from build123d import *

# Parameters (mm, degrees)
BOSS_EXTRUDE4_DEPTH = 200
CUT_EXTRUDE3_START  = -150
CUT_EXTRUDE3_DEPTH  = 150
SKETCH6_R           = 22.5
CUT_EXTRUDE5_DEPTH  = 120
SKETCH7_R           = 32.5
CUT_EXTRUDE6_DEPTH  = 80
FILLET2_R           = 4
SKETCH8_W           = 40
SKETCH8_H           = 40
CUT_EXTRUDE7_DEPTH  = 18
FILLET3_R           = 5
SKETCH10_W          = 10
SKETCH10_H          = 40
CUT_EXTRUDE9_DEPTH  = 69
SKETCH11_R          = 5
CUT_EXTRUDE10_DEPTH = 10


with BuildPart() as part:
    # Sketch1 → Boss-Extrude4 (new body)
    with BuildSketch(Plane(origin=(0, 0, 0), x_dir=(1, 0, 0), z_dir=(0, 1, 0))):
        with BuildLine():
            Line((0, 50), (-25, 50))
            Line((-25, 50), (-25, 31.224990005))
            ThreePointArc((-25, 31.224990005), (0, -40.00000001), (25, 31.224990005))
            Line((25, 31.224990005), (25, 50))
            Line((25, 50), (0, 50))
        make_face()
    extrude(amount=-BOSS_EXTRUDE4_DEPTH)

    # Sketch5 → Cut-Extrude3 (cut)
    with BuildSketch(Plane.XZ.offset(200).offset(CUT_EXTRUDE3_START)):
        with BuildLine():
            Line((-25, -31.224990005), (-25, -50))
            Line((-25, -50), (25, -50))
            Line((25, -50), (25, -31.224990005))
            ThreePointArc((25, -31.224990005), (0, -40.00000001), (-25, -31.224990005))
        make_face()
    extrude(amount=CUT_EXTRUDE3_DEPTH, mode=Mode.SUBTRACT)

    # Sketch6 → Cut-Extrude5 (cut)
    with BuildSketch(Plane(origin=(0, 0, 0), x_dir=(1, 0, 0), z_dir=(0, 1, 0))):
        with Locations(Location((0, 0, 0), (0, 0, 270))):
            Circle(SKETCH6_R)
    extrude(amount=-CUT_EXTRUDE5_DEPTH, mode=Mode.SUBTRACT)

    # Sketch7 → Cut-Extrude6 (cut)
    with BuildSketch(Plane.XZ.offset(200)):
        with Locations(Location((0, 0, 0), (0, 0, 270))):
            Circle(SKETCH7_R)
    extrude(amount=-CUT_EXTRUDE6_DEPTH, mode=Mode.SUBTRACT)

    # Fillet2
    fillet2_edges = [part.edges().sort_by_distance(p)[0] for p in [
        (0, -120, 32.5),
    ]]
    fillet(fillet2_edges, radius=FILLET2_R)

    # Sketch8 → Cut-Extrude7 (cut)
    with BuildSketch(Plane(origin=(0, 0, -50), x_dir=(-1, 0, 0), z_dir=(0, 0, -1))):
        with Locations((0, -25)):
            Rectangle(SKETCH8_W, SKETCH8_H)
    extrude(amount=-CUT_EXTRUDE7_DEPTH, mode=Mode.SUBTRACT)

    # Fillet3
    fillet3_edges = [part.edges().sort_by_distance(p)[0] for p in [
        (20, -45, -41),
        (20, -5, -41),
        (-20, -5, -41),
        (-20, -45, -41),
    ]]
    fillet(fillet3_edges, radius=FILLET3_R)

    # Sketch10 → Cut-Extrude9 (cut)
    with BuildSketch(Plane(origin=(0, 0, 0), x_dir=(0, 0, -1), z_dir=(1, 0, 0))):
        with Locations((0, -165)):
            Rectangle(SKETCH10_W, SKETCH10_H)
        with BuildLine():
            Line((5, -145), (-5, -145))
            ThreePointArc((-5, -145), (0, -140), (5, -145))
        make_face()
        with BuildLine():
            ThreePointArc((5, -185), (0, -190), (-5, -185))
            Line((-5, -185), (5, -185))
        make_face()
    extrude(amount=CUT_EXTRUDE9_DEPTH, mode=Mode.SUBTRACT)

    # Sketch11 → Cut-Extrude10 (cut)
    with BuildSketch(Plane(origin=(0, 0, 0), x_dir=(1, 0, 0), z_dir=(0, 1, 0))):
        with Locations(Location((30, 0, 0), (0, 0, 270))):
            Circle(SKETCH11_R)
        with Locations(Location((21.213203436, -21.213203436, 0), (0, 0, 270))):
            Circle(SKETCH11_R)
        with Locations(Location((0, -30, 0), (0, 0, 270))):
            Circle(SKETCH11_R)
        with Locations(Location((-21.213203436, -21.213203436, 0), (0, 0, 270))):
            Circle(SKETCH11_R)
        with Locations(Location((-30, 0, 0), (0, 0, 270))):
            Circle(SKETCH11_R)
        with Locations(Location((-21.213203436, 21.213203436, 0), (0, 0, 270))):
            Circle(SKETCH11_R)
        with Locations(Location((0, 30, 0), (0, 0, 270))):
            Circle(SKETCH11_R)
        with Locations(Location((21.213203436, 21.213203436, 0), (0, 0, 270))):
            Circle(SKETCH11_R)
    extrude(amount=-CUT_EXTRUDE10_DEPTH, mode=Mode.SUBTRACT)


solid = part.part
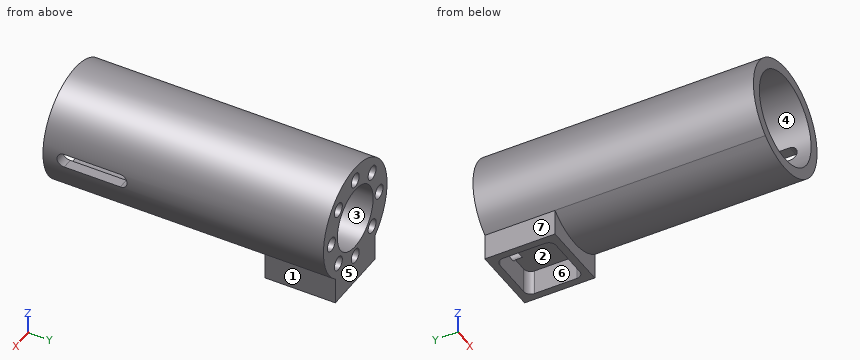
Input: part model. Units: mm. Frame: model coordinates. Face numbers are marked on the shaded views. A direction names the side the tool comes from. Coordinates: 2 decimals unless noted, no trailing zeros. Write each loop counter-clockwise with the first axis right and the second up, starting at its lowest first coordinate (ties: lowest second). Pieces come first, ordered by that corner, then holes. Notation, with made-up numbers: M 79,1 L 105,1 A17 ccw 105,21 Z; hole C 33.25,-7.5 d4. An arc over 180 degrees is marked long. Answer as a JSON object with one key per item and string values. Group by question number.
(1) Ray query, line 1 along X through (y, z) = (-5, 0); line 2 along Y through (x, z) = (25.5, 10); line 3 along Z through (x, y) = (-0.5, -90). Return the intervals inside material, ascending. Write a range as [from, to].
(2) Section D-D on y = -92.5. Output: boundary loops of the cut face in (x, z) (3 decimals).
(3) Contact query for flat-ended pins moving along their axis: P1, Ø6, axis at x = -30, z = 0, coming from the +Y side; P2, Ø1.5, axis at y = -93.5, z = 13, coming from the +X side; P3, Ø4, axis at x = 34.5, y = -169, coming from the -Z side. Output: stop coordinate, or through.
(4) Section C-C on y = -153.5. Output: boundary loops of the cut face in (x, z) (3 decimals).
(5) Section B-B on y = -21.5. Output: boundary loops of the cut face in (x, z) (3 decimals).
(6) Set-up query: the marked faces 1, 2, 3 and 4. Return all of +Z, -Z, +X, -X, +Y, -Y with unobstructed straight access to the full face (end or side cutting, diameter ignored); none if empty.
(7) Section A-A on z = 0. Output: boundary loops of the cut face in (x, y), plus the area to 3 significant figures.
(8) Mould query, pull axis Y, two halves, no side actions, for the marked faces 5, 6 and 7. Classes: pulls with the +Y half, pulls with the -Y half, needs draft (parallel to the pull), parting line crosses it, or undercut.
Result set:
{
 "1": {"line 1": "x = [-40, -35], [-25, -22.5], [22.5, 25], [35, 40]", "line 2": "y = [-120, 0]", "line 3": "z = [-40, -22.49], [22.49, 40]"},
 "2": {"outline": "C 0,0 d80; hole C 0,0 d45"},
 "3": {"P1": "stops at y = -10", "P2": "stops at x = 38.08", "P3": "stops at z = -23.32"},
 "4": {"outline": "M 32.113,-5 A32.5 cw long 32.113,5 L 39.686,5 A40 ccw long 39.686,-5 Z"},
 "5": {"outline": "M -25,-50 L -20,-50 L -20,-32 L 20,-32 L 20,-50 L 25,-50 L 25,-31.225 A40 ccw long -25,-31.225 Z; hole C 0,0 d45"},
 "6": {"face 1": "-Z, +X, +Y, -Y", "face 2": "-Z", "face 3": "+Y, -Y", "face 4": "-Y"},
 "7": {"outline": "M -40,-200 L -32.5,-200 L -32.5,-124 A4 cw -28.5,-120 L -22.5,-120 L -22.5,0 L -25,0 L -25,-10 L -35,-10 L -35,0 L -40,0 Z; M 22.5,-120 L 28.5,-120 A4 cw 32.5,-124 L 32.5,-140 L 40,-140 L 40,0 L 35,0 L 35,-10 L 25,-10 L 25,0 L 22.5,0 Z; M 32.5,-200 L 40,-200 L 40,-190 L 32.5,-190 Z", "area": "4,830 mm2"},
 "8": {"face 5": "pulls with the +Y half", "face 6": "undercut", "face 7": "needs draft"}
}
